```python
from build123d import *

# Parameters (mm, degrees)
SKETCH3_W           = 10
SKETCH3_H           = 5
BOSS_EXTRUDE1_DEPTH = 3
BOSS_EXTRUDE2_DEPTH = 3
CUT_EXTRUDE1_DEPTH  = 4
SKETCH6_R           = 10
CUT_EXTRUDE2_DEPTH  = 4


with BuildPart() as part:
    # Sketch3 → Boss-Extrude1 (new body)
    with BuildSketch(Plane.XY):
        Polygon((0, 0), (54.4906896, 75), (-54.4906896, 75), align=None)
        with Locations((0, 30)):
            Rectangle(SKETCH3_W, SKETCH3_H, mode=Mode.SUBTRACT)
    extrude(amount=BOSS_EXTRUDE1_DEPTH)

    # Sketch4 → Boss-Extrude2 (add)
    with BuildSketch(Plane(origin=(0, 0, 0), x_dir=(-1, 0, 0), z_dir=(0, 0, -1))):
        Polygon((-54.4906896, 75), (-65.38882752, 90), (65.38882752, 90), (54.4906896, 75), align=None)
    extrude(amount=-BOSS_EXTRUDE2_DEPTH)

    # Sketch5 → Cut-Extrude1 (cut, through all)
    with BuildSketch(Plane.XY.offset(3)):
        Polygon((-65.38882752, 90), (-21.79627584, 90), (-43.59255168, 60), align=None)
        Polygon((65.38882752, 90), (21.79627584, 90), (43.59255168, 60), align=None)
    extrude(amount=-CUT_EXTRUDE1_DEPTH, mode=Mode.SUBTRACT)

    # Sketch6 → Cut-Extrude2 (cut, through all)
    with BuildSketch(Plane(origin=(0, 0, 0), x_dir=(-1, 0, 0), z_dir=(0, 0, -1))):
        Circle(SKETCH6_R)
    extrude(amount=-CUT_EXTRUDE2_DEPTH, mode=Mode.SUBTRACT)


solid = part.part
```
Here's how the part is built. I have some questions about the finished solid (model axes, mm). A direction names the side the tool comes from. Round coordinates to 2 decimals unless told otherwise and drop trailing zeros. Loops run counter-clockwise (first coordinate to the right, second up) from the corner with the lowest first, then second, coordinate; pieces in that order, holes last.
1. Suppose I cut it at D-D, the plane x = 36.5. Please give me the cut outline in (y, z), and give its area (3 significant figures).
Answers:
outline: (50.24, 0) - (69.76, 0) - (69.76, 3) - (50.24, 3) - close
area: 58.6 mm2
2. For faces 5 (the face through (5, 30, 1)), 6 (the face through (-32.54, 75.21, 1.52)), which set-ups out of +Z, -Z, +X, -X, +Y, -Y let a thin tool reach every point of the face, with its end or its side?
Answers:
face 5: +Z, -Z
face 6: +Z, -Z, -X, +Y
3. Suppose I cut it at B-B, the plane x = 1. Please give me the cut outline in (y, z).
Answers:
outline: (9.95, 0) - (27.5, 0) - (27.5, 3) - (9.95, 3) - close; (32.5, 0) - (90, 0) - (90, 3) - (32.5, 3) - close
4. Thinking about a two-plate mould opening in Y: for faces 1 (the face through (-5, 30, 1)), 2 (the face through (32.54, 75.21, 1.52)), 3 (the face through (-1, 59, 0)), 4 (the face through (24.47, 33.68, 1.48)), which applies, released by +Y, released by -Y, zero draft, split by the parting line, or undercut?
Answers:
face 1: undercut
face 2: released by +Y
face 3: zero draft
face 4: released by -Y
5. Suppose I cut it at A-A, the plane z = 1. Please give me the cut outline in (x, y).
Answers:
outline: (-43.59, 60) - (-5.88, 8.09) arc R10 cw to (5.88, 8.09) - (43.59, 60) - (21.8, 90) - (-21.8, 90) - close; hole (-5, 27.5) - (5, 27.5) - (5, 32.5) - (-5, 32.5) - close
6. If I drill on probe 1 along X at (y, z) = (30, 1.15); probe 2 along X at (y, z) = (32, 2.1); probe 3 along Y at (x, z) = (-2, 2.05), over which ranges is the centre line in solid material (lowest first)?
Answers:
probe 1: x = -21.8 to -5, 5 to 21.8
probe 2: x = -23.25 to -5, 5 to 23.25
probe 3: y = 9.8 to 27.5, 32.5 to 90
7. Suppose I cut it at C-C, the plane y = 72. Please give me the cut outline in (x, z), and give its area (3 significant figures).
Answers:
outline: (-34.87, 0) - (34.87, 0) - (34.87, 3) - (-34.87, 3) - close
area: 209 mm2
8. Will these pins go through, and if not, where does the flat tip stop? pin 1 (1.5 mm diameter, centred on y = 30.5, z = 1.5, fed in from +X); pin 2 (1.5 mm diameter, centred on y = 29.5, z = 1, fed in from -X); pin 3 (1.5 mm diameter, centred on y = 77.5, z = 2.5, fed in from -X).
Answers:
pin 1: stops at x = 22.7
pin 2: stops at x = -21.98
pin 3: stops at x = -31.42
